Here's how the part is built. I have some questions about the finished solid (model axes, mm). Coordinates: 2 decimals unless noted, no trailing zeros. Use a Markdown table: item, result.
Autodesk Inventor part; units mm, degrees
ref_plane "Start Plane" through (0, 0, 0) normal (0, 0, 1) x (1, 0, 0)
ref_plane "End Plane" through (0, 0, 20) normal (0, 0, 1) x (1, 0, 0)
ref_plane "YZ Plane" through (0, 0, 0) normal (1, 0, 0) x (0, 1, 0)
ref_plane "Start Plane" through (0, 0, 0) normal (0, 0, 1) x (1, 0, 0)
ref_plane "End Plane" through (0, 0, 20) normal (0, 0, 1) x (1, 0, 0)
sketch "Sketch1" plane through (0, 0, 0) normal (0, 0, 1) x (1, 0, 0)
  line L0 (10, -4.5951) -> (10, -8.2)
  line L1 (-10, -8.2) -> (-10, -4.5951)
  line L2 (-10, 10) -> (10, -10) construction
  line L3 (10, 10) -> (-10, -10) construction
  circle A0 centre (0, 0) radius 2.1
  line L4 (-2.84, -3.9007) -> (2.84, -3.9007)
  line L5 (3.9007, -2.84) -> (3.9007, 2.84)
  line L6 (2.84, 3.9007) -> (-2.84, 3.9007)
  line L7 (-3.9007, 2.84) -> (-3.9007, -2.84)
  line L8 (-3.9007, -3.9007) -> (3.9007, 3.9007) construction
  line L9 (3.9007, -3.9007) -> (-3.9007, 3.9007) construction
  line L10 (-3.9007, -2.84) -> (-2.84, -3.9007) construction
  line L11 (-2.84, -3.9007) -> (-5.4993, -6.56)
  line L12 (-5.4993, -6.56) -> (-5.4993, -8.2)
  line L13 (-5.4993, -8.2) -> (-2.7951, -8.2)
  line L14 (-2.7951, -8.2) -> (-4.5951, -10)
  line L15 (0, 0) -> (0, -3.9007) construction
  line L16 (3.9007, -2.84) -> (2.84, -3.9007) construction
  line L17 (2.84, -3.9007) -> (5.4993, -6.56)
  line L18 (5.4993, -6.56) -> (5.4993, -8.2)
  line L19 (5.4993, -8.2) -> (2.7951, -8.2)
  line L20 (2.7951, -8.2) -> (4.5951, -10)
  line L21 (-2.84, -3.9007) -> (-3.9007, -2.84) construction
  line L22 (-3.9007, -2.84) -> (-6.56, -5.4993)
  line L23 (-6.56, -5.4993) -> (-8.2, -5.4993)
  line L24 (-8.2, -5.4993) -> (-8.2, -2.7951)
  line L25 (-8.2, -2.7951) -> (-10, -4.5951)
  line L26 (3.9007, -2.84) -> (6.56, -5.4993)
  line L27 (6.56, -5.4993) -> (8.2, -5.4993)
  line L28 (8.2, -5.4993) -> (8.2, -2.7951)
  line L29 (8.2, -2.7951) -> (10, -4.5951)
  arc A1 (-10, -8.2) -> (-8.2, -10) centre (-8.2, -8.2) ccw
  arc A2 (8.2, -10) -> (10, -8.2) centre (8.2, -8.2) ccw
  line L30 (-8.2, -6.56) -> (-7.7111, -6.56)
  line L31 (-6.6505, -8.2) -> (-8.2, -8.2)
  line L32 (-8.2, -8.2) -> (-8.2, -6.56)
  line L33 (-6.6505, -7.6207) -> (-7.7111, -6.56)
  line L34 (-6.6505, -7.6207) -> (-6.6505, -8.2)
  line L35 (8.2, -6.56) -> (7.7111, -6.56)
  line L36 (6.6505, -8.2) -> (8.2, -8.2)
  line L37 (8.2, -8.2) -> (8.2, -6.56)
  line L38 (6.6505, -7.6207) -> (7.7111, -6.56)
  line L39 (6.6505, -7.6207) -> (6.6505, -8.2)
  line L40 (8.2, -10) -> (4.5951, -10)
  line L41 (-4.5951, -10) -> (-8.2, -10)
  line L42 (-3.9007, 0) -> (3.9007, 0) construction
  line L43 (10, 4.5951) -> (10, 8.2)
  line L44 (-10, 8.2) -> (-10, 4.5951)
  line L45 (-2.84, 3.9007) -> (2.84, 3.9007)
  line L46 (-3.9007, 2.84) -> (-2.84, 3.9007) construction
  line L47 (-2.84, 3.9007) -> (-5.4993, 6.56)
  line L48 (-5.4993, 6.56) -> (-5.4993, 8.2)
  line L49 (-5.4993, 8.2) -> (-2.7951, 8.2)
  line L50 (-2.7951, 8.2) -> (-4.5951, 10)
  line L51 (2.84, 3.9007) -> (5.4993, 6.56)
  line L52 (5.4993, 6.56) -> (5.4993, 8.2)
  line L53 (5.4993, 8.2) -> (2.7951, 8.2)
  line L54 (2.7951, 8.2) -> (4.5951, 10)
  line L55 (3.9007, 2.84) -> (2.84, 3.9007) construction
  line L56 (-8.2, 2.7951) -> (-10, 4.5951)
  line L57 (-2.84, 3.9007) -> (-3.9007, 2.84) construction
  line L58 (-3.9007, 2.84) -> (-6.56, 5.4993)
  line L59 (-6.56, 5.4993) -> (-8.2, 5.4993)
  line L60 (-8.2, 5.4993) -> (-8.2, 2.7951)
  line L61 (3.9007, 2.84) -> (6.56, 5.4993)
  line L62 (6.56, 5.4993) -> (8.2, 5.4993)
  line L63 (8.2, 5.4993) -> (8.2, 2.7951)
  line L64 (8.2, 2.7951) -> (10, 4.5951)
  arc A3 (-8.2, 10) -> (-10, 8.2) centre (-8.2, 8.2) ccw
  arc A4 (10, 8.2) -> (8.2, 10) centre (8.2, 8.2) ccw
  line L65 (-8.2, 6.56) -> (-7.7111, 6.56)
  line L66 (-6.6505, 8.2) -> (-8.2, 8.2)
  line L67 (-8.2, 8.2) -> (-8.2, 6.56)
  line L68 (-6.6505, 7.6207) -> (-7.7111, 6.56)
  line L69 (-6.6505, 7.6207) -> (-6.6505, 8.2)
  line L70 (8.2, 6.56) -> (7.7111, 6.56)
  line L71 (6.6505, 7.6207) -> (7.7111, 6.56)
  line L72 (8.2, 8.2) -> (8.2, 6.56)
  line L73 (6.6505, 7.6207) -> (6.6505, 8.2)
  line L74 (6.6505, 8.2) -> (8.2, 8.2)
  line L75 (8.2, 10) -> (4.5951, 10)
  line L76 (-4.5951, 10) -> (-8.2, 10)
  line L77 (-8.2, 10) -> (-4.5951, 10)
  line L78 (4.5951, 10) -> (8.2, 10)
  point P0 (8.2, -8.2)
  point P1 (0, 3.9007)
  point P2 (8.2, 8.2)
  dimension "Width" = 20
  dimension "Height" = 20
  dimension "d2" = 4.2
  dimension "d3" = 1.5
  dimension "d4" = 1.64
  dimension "d6" = 5.68
  dimension "d7" = 1.8
  dimension "d9" = 1.5
extrude "Body" add sketch "Sketch1" along normal blind 500
sketch "Sketch4" plane through (0, 0, 0) normal (0, 0, 1) x (1, 0, 0)
  line L0 (0, 0) -> (10, 0)
ref_plane "Work Plane4" through (0, 0, 0) normal (0, -1, 0) x (1, 0, 0)
sketch "Sketch5" plane through (0, 0, 0) normal (0, -1, 0) x (1, 0, 0)
  line L0 (-2, 0) -> (12, 0) construction
  line L1 (-2, 20) -> (12, 20) construction
  dimension "d17" = 20
equation "\"G_OFFSET_START\" = 0"
equation "\"G_OFFSET_END\" = 0"
equation "\"G_L\" = d17"
properties part number "V-slot 20 mm x 20 mm" material "Aluminum 6061"
Q1. Will these pins go through, and if not, where does the flat tip stop? P1, Ø3, axis at x = 0, z = 147, coming from the +Y side; P2, Ø1, axis at x = 7, y = 6, coming from the -Z side; P3, Ø3, axis at y = -3, z = 147, coming from the +X side; P4, Ø6, axis at x = 1, z = 162, coming from the -Y side.
Check values:
| item | result |
|---|---|
| P1 | y = 3.9 |
| P2 | z = 0 |
| P3 | x = 9.9 |
| P4 | y = -9.4 |
Q2. Please list where these lines run through material, in increasing order: L1, parallel to X at y = 7.75, z = 380.5; L2, parallel to Y at x = 0, z = 267.5; L3, parallel to X at y = -3, z = 26. Write a range as from..to.
Check values:
| item | result |
|---|---|
| L1 | -10..-8.2, -6.65..-5.5, 5.5..6.65, 8.2..10 |
| L2 | -3.9..-2.1, 2.1..3.9 |
| L3 | -8.4..-8.2, -4.06..4.06, 8.2..8.4 |
Q3. I want a section at A-A, the plane z = 246.5. Give the number of separate pieces and of enclosed holes in the cut face, then the cut area to 3 significant figures.
Check values:
| item | result |
|---|---|
| separate pieces | 1 |
| enclosed holes | 5 |
| area | 161 mm^2 |
